from build123d import *

# Parameters (mm, degrees)
SKETCH1_R           = 1.778
SKETCH1_R_2         = 1.7653
BOSS_EXTRUDE1_DEPTH = 5.842
FILLET3_R           = 1.5875
FILLET6_R           = 6.35
FILLET7_R           = 0.396875
FILLET9_R           = 0.79375


with BuildPart() as part:
    # Sketch1 → Boss-Extrude1 (new body)
    # profile 1 of 2: a face of its own
    with BuildSketch(Plane(origin=(0, 0, 0), x_dir=(1, 0, 0), z_dir=(0, 1, 0))):
        with BuildLine():
            ThreePointArc((4.7625, 0), (3.367596045, -3.367596045), (0, -4.7625))
            Line((0, -4.7625), (0, -21.43125))
            Line((0, -21.43125), (-4.7625, -21.43125))
            Line((-4.7625, -21.43125), (-4.7625, -38.1))
            Line((-4.7625, -38.1), (0, -38.1))
            ThreePointArc((0, -38.1), (18.016692001, -33.570951868), (31.75, -21.060567419))
            Line((31.75, -21.060567419), (28.442708333, -18.866758313))
            Line((28.442708333, -18.866758313), (30.197755618, -16.220924979))
            Line((30.197755618, -16.220924979), (20.130923816, -9.543344196))
            Line((20.130923816, -9.543344196), (20.98465671, -8.204646532))
            Line((20.98465671, -8.204646532), (2.632570927, 3.96875))
            ThreePointArc((2.632570927, 3.96875), (4.196368984, 2.2520865), (4.7625, 0))
        make_face()
        with Locations(Location((6.35, -24.593444248, 0), (0, 0, 270))):
            Circle(SKETCH1_R, mode=Mode.SUBTRACT)
    # profile 2 of 2: a face of its own
    with BuildSketch(Plane(origin=(0, 0, 0), x_dir=(1, 0, 0), z_dir=(0, 1, 0))):
        with BuildLine():
            ThreePointArc((4.7625, 0), (3.367596045, -3.367596045), (0, -4.7625))
            ThreePointArc((0, -4.7625), (-3.367596045, 3.367596045), (4.7625, 0))
        make_face()
        with Locations(Location((0, 0, 0), (0, 0, 270))):
            Circle(SKETCH1_R_2, mode=Mode.SUBTRACT)
    extrude(amount=BOSS_EXTRUDE1_DEPTH)

    # Fillet3
    fillet3_edges = [part.edges().sort_by_distance(p)[0] for p in [
        (-4.7625, 2.921, 38.1),
        (-4.7625, 2.921, 21.43125),
        (0, 2.921, 21.43125),
    ]]
    fillet(fillet3_edges, radius=FILLET3_R)

    # Fillet6
    fillet6_edges = [part.edges().sort_by_distance(p)[0] for p in [
        (0, 2.921, 4.7625),
    ]]
    fillet(fillet6_edges, radius=FILLET6_R)

    # Fillet7
    fillet7_edges = [part.edges().sort_by_distance(p)[0] for p in [
        (30.197755618, 2.921, 16.220924979),
        (31.75, 2.921, 21.060567419),
    ]]
    fillet(fillet7_edges, radius=FILLET7_R)

    # Fillet9
    fillet9_edges = [part.edges().sort_by_distance(p)[0] for p in [
        (20.98465671, 2.921, 8.204646532),
        (20.130923816, 2.921, 9.543344196),
    ]]
    fillet(fillet9_edges, radius=FILLET9_R)


solid = part.part
Could you check a few things on this model? Use its own coordinates, in mm. A direction names the side the tool comes from. Coordinates: 2 decimals unless noted, no trailing zeros. Loops run counter-clockwise (first coordinate to the right, second up) from the corner with the lowest first, then second, coordinate; pieces in that order, holes last.
1. Imagine slicing it at C-C (x = 6.35). Please give me the cut outline in (y, z), and give its area (3 significant figures).
2. Imagine slicing it at D-D (z = 5). Please give me the cut outline in (x, y), and give its area (3 significant figures).
3. We'd pull the mould along X, two halves only. Please class faces 1 (the face through (11.608, 2.88, 1.985)), 2 (the face through (0, 3, 14)), 3 (the face through (-1.723, 2.88, -0.383)), 4 (the face through (6.88, 2.88, 26.29)): released by +X, released by -X, zero draft, split by the parting line, or undercut.
4. Imagine slicing it at A-A (z = 25). Please give me the cut outline in (x, y).
5. Imagine slicing it at B-B (y = 1.25). Give the number of separate pieces and of enclosed holes in the cut face, and give its area (3 significant figures).
6. For faces 5 (the face through (-4.3, 3, 21.9)), 6 (the face through (-3.996, 2.88, -2.591)), 7 (the face through (30, 2.9, 19.9)), which set-ups out of +Z, -Z, +X, -X, +Y, -Y let a thin tool reach every point of the face, with its end or its side?
7. I need wall thicknesses on L1, parallel to Z at x = -1.5, y = 1.1; L2, parallel to X at y = 1.7, z = 16; L3, parallel to Z at x = 29.5, y = 2. Which ranges of each line are inside material? Lowest first, please.
8. For P1, Ø0.5, axis at x = -3, y = 3, coming from the -Z side; P2, Ø3, axis at x = 13.5, y = 2, coming from the +Z side; P3, Ø3, axis at y = 2, z = 13.5, coming from the -X side, each with a flat end and sliding along its axis, tell me the tip position at first contact or that it passes through.
Computed values:
1. outline: (0, -1.5) - (5.84, -1.5) - (5.84, 22.82) - (0, 22.82) - close; (0, 26.37) - (5.84, 26.37) - (5.84, 37.57) - (0, 37.57) - close
1. area: 207 mm2
2. outline: (-1.52, 0) - (16.15, 0) - (16.15, 5.84) - (-1.52, 5.84) - close
2. area: 103 mm2
3. face 1: released by +X
3. face 2: released by -X
3. face 3: undercut
3. face 4: undercut
4. outline: (-4.76, 0) - (4.62, 0) - (4.62, 5.84) - (-4.76, 5.84) - close; (8.08, 0) - (28.75, 0) - (28.75, 5.84) - (8.08, 5.84) - close
5. separate pieces: 1
5. enclosed holes: 2
5. area: 962 mm2
6. face 5: -X, +Y, -Y
6. face 6: +Y, -Y
6. face 7: +X, +Y, -Y
7. L1: z = -4.52 to -0.93, 0.93 to 5.02, 21.43 to 38.1
7. L2: x = 0 to 29.86
7. L3: z = 15.76 to 17.27, 19.57 to 24.11
8. P1: stops at z = -3.89
8. P2: stops at z = 36.16
8. P3: stops at x = 0
